Can you work these out from the model? Positions are in its coordinate system, mm. A direction names the side the tool comes from. Give positions to 0.01 mm unless a question says otherwise; leave off trailing zeros. Loops run counter-clockwise (first coordinate to the right, second up) from the corner with the lowest first, then second, coordinate; pieces in that order, holes last.
from build123d import *

# Parameters (mm, degrees)
SKETCH1_R           = 1.7145
BOSS_EXTRUDE1_DEPTH = 42.0878
BOSS_EXTRUDE2_DEPTH = 2.7686
SKETCH3_R           = 1.7018
BOSS_EXTRUDE3_DEPTH = 7.3152
SKETCH4_R           = 1.7018
SKETCH4_R_2         = 1.651
CUT_EXTRUDE1_DEPTH  = 5.969
SKETCH5_R           = 1.7145
SKETCH5_R_2         = 1.6637
CUT_EXTRUDE2_DEPTH  = 14.859


with BuildPart() as part:
    # Sketch1 → Boss-Extrude1 (new body)
    with BuildSketch(Plane(origin=(0, 0, 0), x_dir=(1, 0, 0), z_dir=(0, 1, 0))):
        with Locations(Location((0, 0, 0), (0, 0, 270))):  # turned: the seam where the file's is
            Circle(SKETCH1_R)
    extrude(amount=-BOSS_EXTRUDE1_DEPTH)

    # Sketch2 → Boss-Extrude2 (add)
    with BuildSketch(Plane(origin=(0, 0, 0), x_dir=(1, 0, 0), z_dir=(0, 1, 0))):
        Polygon((1.844793874, 3.195276719), (-1.844793874, 3.195276719), (-3.689587747, 0), (-1.844793874, -3.195276719), (1.844793874, -3.195276719), (3.689587747, 0), align=None)
    extrude(amount=BOSS_EXTRUDE2_DEPTH)

    # Sketch3 → Boss-Extrude3 (add)
    with BuildSketch(Plane(origin=(0, 2.7686, 0), x_dir=(1, 0, 0), z_dir=(0, 1, 0))):
        with Locations(Location((0, 0, 0), (0, 0, 270))):  # turned: the seam where the file's is
            Circle(SKETCH3_R)
    extrude(amount=BOSS_EXTRUDE3_DEPTH)

    # Sketch4 → Cut-Extrude1 (cut)
    with BuildSketch(Plane(origin=(0, 10.0838, 0), x_dir=(1, 0, 0), z_dir=(0, 1, 0))):
        with Locations(Location((0, 0, 0), (0, 0, 270))):  # turned: the seam where the file's is
            Circle(SKETCH4_R)
        with Locations(Location((0, 0, 0), (0, 0, 270))):  # turned: the seam where the file's is
            Circle(SKETCH4_R_2, mode=Mode.SUBTRACT)
    extrude(amount=-CUT_EXTRUDE1_DEPTH, mode=Mode.SUBTRACT)

    # Sketch5 → Cut-Extrude2 (cut)
    with BuildSketch(Plane.XZ.offset(42.0878)):
        with Locations(Location((0, 0, 0), (0, 0, 90))):  # turned: the seam where the file's is
            Circle(SKETCH5_R)
        with Locations(Location((0, 0, 0), (0, 0, 270))):  # turned: the seam where the file's is
            Circle(SKETCH5_R_2, mode=Mode.SUBTRACT)
    extrude(amount=-CUT_EXTRUDE2_DEPTH, mode=Mode.SUBTRACT)


solid = part.part
(1) Suppose I cut it at A-A on x = 0. List the corners of the cut face in (y, z) for me.
Returned:
outline: (-42.09, -1.66) - (-27.23, -1.66) - (-27.23, -1.71) - (0, -1.71) - (0, -3.2) - (2.77, -3.2) - (2.77, -1.7) - (4.11, -1.7) - (4.11, -1.65) - (10.08, -1.65) - (10.08, 1.65) - (4.11, 1.65) - (4.11, 1.7) - (2.77, 1.7) - (2.77, 3.2) - (0, 3.2) - (0, 1.71) - (-27.23, 1.71) - (-27.23, 1.66) - (-42.09, 1.66) - close
(2) Please list where these lines run through material, in increasing order: probe 1 along Y at (x, z) = (-0.25, -2); probe 2 along X at (y, z) = (-14.5, 0); probe 3 along Z at (x, y) = (-0.5, -31.5).
Returned:
probe 1: y = 0 to 2.77
probe 2: x = -1.71 to 1.71
probe 3: z = -1.59 to 1.59
(3) Suppose I cut it at C-C on y = 3.5. List the corners of the cut face in (x, z) for me.
Returned:
outline: circle Ø3.4 at (0, 0)
(4) Will these pins go through, and if not, where does the flat tip stop? P1, Ø2, axis at x = 0.5, y = -30, coming from the +Z side; P2, Ø1.5, axis at y = -8.5, z = -2, coming from the -X side; P3, Ø1, axis at y = -7, z = -1, coming from the -X side.
Returned:
P1: stops at z = 1.66
P2: stops at x = -1.17
P3: stops at x = -1.64
(5) Which directions (+Z, -Z, +X, -X, +Y, -Y) give clear straight access to the entire face, cutting with the end or side of a thin tool? Please do faces 1 (the flat face through (-2.78, 1.365, 1.575)), 2 (the cylindrical face through (-1.624, -34.762, 0.361)), 3 (the flat face through (2, 2.769, -1)).
Returned:
face 1: +Z, -X, +Y, -Y
face 2: -Y
face 3: +Y
(6) Suppose I cut it at B-B on z = -0.5. List the corners of the cut face in (x, y) for me.
Returned:
outline: (-3.4, 0) - (-1.64, 0) - (-1.64, -27.23) - (-1.59, -27.23) - (-1.59, -42.09) - (1.59, -42.09) - (1.59, -27.23) - (1.64, -27.23) - (1.64, 0) - (3.4, 0) - (3.4, 2.77) - (1.63, 2.77) - (1.63, 4.11) - (1.57, 4.11) - (1.57, 10.08) - (-1.57, 10.08) - (-1.57, 4.11) - (-1.63, 4.11) - (-1.63, 2.77) - (-3.4, 2.77) - close
(7) Suppose I cut it at D-D on y = -10. List the corners of the cut face in (x, z) for me, plus the area to 3 significant figures.
Returned:
outline: circle Ø3.43 at (0, 0)
area: 9.23 mm2
